The model under review builds one solid part; all positions refer to its coordinate system, in mm. A direction names the side the tool comes from. Round coordinates to 2 decimals unless told otherwise and drop trailing zeros. Order: outer loops, then holes, each group sorted by start corner. A loop starts at its lowest first (then second) coordinate and runs counter-clockwise, first axis right, second up.
```python
from build123d import *

# Parameters (mm, degrees)
F2_T     = -1.25
F3_R     = 2.8299175035
F4_DEPTH = 25


with BuildPart() as f1:
    # F0 (on Front) → F1 (revolve)
    with BuildSketch(Plane.XZ):
        Polygon((0, -12.4857185782), (0, 12.9142814218), (-4, 12.9142814218), (-4, 7.1125508785), (-15, -12.4857185782), align=None)
    revolve(axis=Axis((0, 0, 21.6972688213), (0, 0, -1)))

    # F2
    f2_openings = [f1.faces().sort_by_distance(p)[0] for p in [
        (0, 0, -12.485719),
    ]]
    offset(amount=F2_T, openings=f2_openings, kind=Kind.INTERSECTION)

    # F3 (on face) → F4 (cut)
    with BuildSketch(Plane.XY.offset(12.9142814218)):
        Circle(F3_R)
    extrude(amount=-F4_DEPTH, mode=Mode.SUBTRACT)


solid = f1.part
```
(1) To check wall thickness, follow probe 1 along Y at (x, z) = (0, 9); probe 2 along X at (y, z) = (0, -9); probe 3 along X at (y, z) = (2.25, -8.5). State the ranges of each line that lie inside material, in increasing order.
Data:
probe 1: y = -4 to -2.83, 2.83 to 4
probe 2: x = -13.04 to -11.61, 11.61 to 13.04
probe 3: x = -12.56 to -11.1, 11.1 to 12.56
(2) For faces 5 (the flat face through (1, 3, 12.914)), 6 (the cylindrical face through (0.867, -3.905, 9.973)), list the 3-axis set-ups (+Z, -Z, +X, -X, +Y, -Y) from which the entire face can be reached by the end or side of a thin tool; tool diameter is ignored.
Data:
face 5: +Z, +X, -X, +Y, -Y
face 6: +Z
(3) Consider section C-C (z = 11.75). Write out the cut boundary in (x, y), and give its area (3 significant figures).
Data:
outline: circle Ø8 at (0, 0); hole circle Ø5.66 at (0, 0)
area: 25.1 mm2
(4) Consider section A-A (x = 0). Write out the cut boundary in (y, z), and give its area (3 significant figures).
Data:
outline: (-15, -12.49) - (-13.57, -12.49) - (-2.83, 6.64) - (-2.83, 12.91) - (-4, 12.91) - (-4, 7.11) - close; (2.83, 6.64) - (13.57, -12.49) - (15, -12.49) - (4, 7.11) - (4, 12.91) - (2.83, 12.91) - close
area: 69.6 mm2
(5) Consider section D-D (z = -2.25). Write out the cut boundary in (x, y), and give its area (3 significant figures).
Data:
outline: circle Ø18.51 at (0, 0); hole circle Ø15.64 at (0, 0)
area: 76.9 mm2
(6) Insertion check: pin 1 (1 mm diameter, centred on x = 7.5, y = 8.5, fed in from -Z); pin 2 (2 mm diameter, centred on x = -8, y = -1.5, fed in from +Z); pin 3 (5 mm diameter, centred on x = -12, z = -5.5, fed in from -Y). Each pin has a flat end and moves straight along its axis. Give the tip position at first contact, or say it passes through.
Data:
pin 1: stops at z = -9.4
pin 2: stops at z = 1.52
pin 3: stops at y = -6.5
(7) Draft analysis for pull direction Y (two halves, no side actions). For faces 1 (the flat face through (3.4, -13.3, -12.486)), 2 (the conical face through (-2.72, -5.22, 1.2)), 3 (the conical face through (1.546, -6.963, 1.531)), 4 (the cylindrical face through (-0.613, -2.763, 9.823)), state which applies: pulls with the +Y half, pulls with the -Y half, needs draft (parallel to the pull), parting line crosses it, or undercut.
Data:
face 1: needs draft
face 2: undercut
face 3: parting line crosses it
face 4: undercut
